Check sheet for the modelled part. Datum: model origin and axes. Units: mm. Round coordinates to 2 decimals unless told otherwise and drop trailing zeros. Order: outer loops, then holes, each group sorted by start corner. A loop starts at its lowest first (then second) coordinate and runs counter-clockwise, first axis right, second up. Notation, with made-up numbers: (56, 59) -> (76, 59) arc R13 cw to (76, 66) -> close; hole circle Ø8 at (50.5, -18.75). An arc over 180 degrees is marked (long way). Answer in a Markdown table with one row per item.
Autodesk Inventor part; units mm, degrees
ref_plane "YZ Plane" through (0, 0, 0) normal (1, 0, 0) x (0, 1, 0)
ref_plane "XZ Plane" through (0, 0, 0) normal (0, 1, 0) x (-1, 0, 0)
ref_plane "XY Plane" through (0, 0, 0) normal (0, 0, 1) x (1, 0, 0)
sketch "Sketch1" plane through (0, 0, 0) normal (0, 1, 0) x (-1, 0, 0)
  line L0 (0, -60) -> (-100, -60)
  line L1 (-100, -60) -> (-100, 0)
  line L2 (-100, 0) -> (0, 0)
  line L3 (0, 0) -> (0, -60)
  dimension "d0" = 100
  dimension "d1" = 60
extrude "Extrusion1" add sketch "Sketch1" along normal blind 3
sketch "Sketch2" plane through (0, 3, 0) normal (0, 1, 0) x (1, 0, 0)
  circle A0 centre (5, 55) radius 1.75
  line L0 (100, 60) -> (0, 60)
  line L1 (0, 60) -> (0, 0)
  circle A1 centre (95, 55) radius 1.75
  circle A2 centre (5, 5) radius 1.75
  circle A3 centre (95, 5) radius 1.75
  circle A4 centre (87.5, 42.5) radius 1.75
  circle A5 centre (87.5, 17.5) radius 1.75
  line L2 (100, 0) -> (100, 60)
  circle A6 centre (49.5, 47) radius 1.75
  circle A7 centre (49.5, 13) radius 1.75
  dimension "d4" = 3.5
  dimension "d5" = 5
  dimension "d6" = 5
  dimension "d9" = 90
  dimension "d12" = 50
  dimension "d15" = 3.5
  dimension "d16" = 3.5
  dimension "d17" = 25
  dimension "d18" = 0
  dimension "d19" = 12.5
  dimension "d20" = 3.5
  dimension "d21" = 3.5
  dimension "d22" = 34
  dimension "d23" = 0
  dimension "d24" = 38
  dimension "d25" = 17.5
  dimension "d26" = 13
extrude "Extrusion2" cut sketch "Sketch2" against normal through all
properties part number "rfid_cover"
Item 1: Cross-section at C-C (z = -47). Record the boundary of the cut face in (x, y), and give its area (4 significant figures).
Result sheet:
| item | result |
|---|---|
| outline | (0, 0) -> (47.75, 0) -> (47.75, 3) -> (0, 3) -> close; (51.25, 0) -> (100, 0) -> (100, 3) -> (51.25, 3) -> close |
| area | 289.5 mm^2 |
Item 2: Scan lines: line 1 (X direction, y = 1.05, z = -5); line 2 (Z direction, x = 5, y = 1.35); line 3 (Z direction, x = 49.5, y = 1.55). Record each from-to range of solid material in increasing order. Write a range as [from, to].
Result sheet:
| item | result |
|---|---|
| line 1 | x = [0, 3.25], [6.75, 93.25], [96.75, 100] |
| line 2 | z = [-60, -56.75], [-53.25, -6.75], [-3.25, 0] |
| line 3 | z = [-60, -48.75], [-45.25, -14.75], [-11.25, 0] |
Item 3: Cross-section at A-A (x = 87.5). Record the boundary of the cut face in (y, z).
Result sheet:
| item | result |
|---|---|
| outline | (0, -60) -> (3, -60) -> (3, -44.25) -> (0, -44.25) -> close; (0, -40.75) -> (3, -40.75) -> (3, -19.25) -> (0, -19.25) -> close; (0, -15.75) -> (3, -15.75) -> (3, 0) -> (0, 0) -> close |
Item 4: Mould release check, pull along Z, two halves, no side actions. Record for faces 1 (the flat face through (100, 1, -30)), 2 (the cylindrical face through (94.62, 1.52, -3.29)), 3 (the flat face through (51, 1, 0)): pulls with the +Z half, pulls with the -Z half, needs draft (parallel to the pull), parting line crosses it, or undercut.
Result sheet:
| item | result |
|---|---|
| face 1 | needs draft |
| face 2 | undercut |
| face 3 | pulls with the +Z half |
Item 5: Cross-section at B-B (z = -55). Record the boundary of the cut face in (x, y).
Result sheet:
| item | result |
|---|---|
| outline | (0, 0) -> (3.25, 0) -> (3.25, 3) -> (0, 3) -> close; (6.75, 0) -> (93.25, 0) -> (93.25, 3) -> (6.75, 3) -> close; (96.75, 0) -> (100, 0) -> (100, 3) -> (96.75, 3) -> close |
